Build history of the part. All positions in model axes, mm. Face numbers are marked on the shaded views. A direction names the side the tool comes from. Coordinates: 2 decimals unless noted, no trailing zeros. Loops run counter-clockwise (first coordinate to the right, second up) from the corner with the lowest first, then second, coordinate; pieces in that order, holes last.
Item 1: Cut at B-B (y = 39). List the corners of the cut face in (x, z), and give its area (3 significant figures).
Item 2: Cut at A-A (x = 39). List the corners of the cut face in (y, z), and give its area (3 significant figures).
Item 3: Flat gauge pins, fed straight in: pin 1 (8 mm diameter, centred on y = -15.5, z = 59.5, fed in from -X); pin 2 (2 mm diameter, centred on x = 15, y = 17, fed in from +Z); pin 3 (8 mm diameter, centred on x = -35.5, z = 77.5, fed in from +Y). Where does each tip first touch, or does it go through?
Item 4: Drill centre lines: line 1 along Z through (x, y) = (-13, 0); line 2 along Y through (x, z) = (-22.5, 70); line 3 along X through (y, z) = (13.5, 57.5). Where is each one in solid material? Low to high.
Item 5: 3-axis set-ups, long thin cutter, end or side, ignore diameter. For the marked faces 1, 2, 3 and 4: which of +Z, -Z, +X, -X, +Y, -Y reach the whole face in a straight line?
Item 6: Cut at C-C (z = 20.5). List the corners of the cut face in (x, y), and give its area (3 significant figures).
from build123d import *

# Parameters (mm, degrees)
F0_W      = 100
F0_H      = 100
F1_DEPTH  = 75
F2_W      = 52.5
F2_H      = 52.5
F3_DEPTH  = 10
F4_W      = 5
F4_H      = 52.5
F5_DEPTH  = 1
F6_W      = 10
F6_H      = 10
F7_DEPTH  = 1
F8_W      = 10
F8_H      = 11
F9_DEPTH  = 1
F10_W     = 10
F10_H     = 3.468894
F11_DEPTH = 1
F12_W     = 10
F12_H     = 3.531106
F13_DEPTH = 1


with BuildPart() as f1:
    # F0 (on Top) → F1 (new body)
    with BuildSketch(Plane.XY):
        with Locations((-0.019781, -0.031106)):
            Rectangle(F0_W, F0_H)
    extrude(amount=F1_DEPTH)

    # F2 (on face) → F3 (join)
    with BuildSketch(Plane.XY.offset(75)):
        with Locations((26.25, 26.25)):
            Rectangle(F2_W, F2_H)
        with Locations((-26.25, 26.25)):
            Rectangle(F2_W, F2_H)
        with Locations((26.25, -26.25)):
            Rectangle(F2_W, F2_H)
        with Locations((-26.25, -26.25)):
            Rectangle(F2_W, F2_H)
    extrude(amount=F3_DEPTH)

    # F4 (on face) → F5 (join)
    with BuildSketch(Plane.XY.offset(85)):
        with Locations((-2.5, -26.25)):
            Rectangle(F4_W, F4_H)
        with Locations((-2.5, 26.25)):
            Rectangle(F4_W, F4_H)
        with Locations((2.5, -26.25)):
            Rectangle(F4_W, F4_H)
        with Locations((2.5, 26.25)):
            Rectangle(F4_W, F4_H)
    extrude(amount=F5_DEPTH)

    # F6 (on face) → F7 (join)
    with BuildSketch(Plane.XZ.offset(52.5)):
        with Locations((0, 80)):
            Rectangle(F6_W, F6_H)
    extrude(amount=F7_DEPTH)

    # F8 (on face) → F9 (join)
    with BuildSketch(Plane(origin=(0, 52.5, 0), x_dir=(-1, 0, 0), z_dir=(0, 1, 0))):
        with Locations((0, 80.5)):
            Rectangle(F8_W, F8_H)
    extrude(amount=F9_DEPTH)

    # F10 (on face) → F11 (join)
    with BuildSketch(Plane(origin=(0, 0, 75), x_dir=(1, 0, 0), z_dir=(0, 0, -1))):
        with Locations((0, 51.765553)):
            Rectangle(F10_W, F10_H)
    extrude(amount=F11_DEPTH)

    # F12 (on face) → F13 (join)
    with BuildSketch(Plane(origin=(0, 0, 75), x_dir=(1, 0, 0), z_dir=(0, 0, -1))):
        with Locations((0, -51.734447)):
            Rectangle(F12_W, F12_H)
    extrude(amount=F13_DEPTH)


solid = f1.part
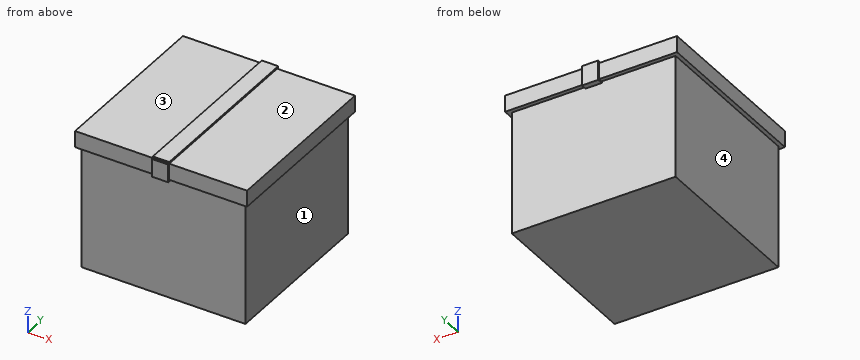
Filled sheet:
1. outline: (-52.5, 75) - (-50.02, 75) - (-50.02, 0) - (49.98, 0) - (49.98, 75) - (52.5, 75) - (52.5, 85) - (5, 85) - (5, 86) - (-5, 86) - (-5, 85) - (-52.5, 85) - close
1. area: 8,560 mm2
2. outline: (-52.5, 75) - (-50.03, 75) - (-50.03, 0) - (49.97, 0) - (49.97, 75) - (52.5, 75) - (52.5, 85) - (-52.5, 85) - close
2. area: 8,550 mm2
3. pin 1: stops at x = -50.02
3. pin 2: stops at z = 85
3. pin 3: stops at y = 52.5
4. line 1: z = 0 to 85
4. line 2: y = -50.03 to 49.97
4. line 3: x = -50.02 to 49.98
5. face 1: -Z, +X, +Y, -Y
5. face 2: +Z, +X, +Y, -Y
5. face 3: +Z, -X, +Y, -Y
5. face 4: -Z, -X, +Y, -Y
6. outline: (-50.02, -50.03) - (49.98, -50.03) - (49.98, 49.97) - (-50.02, 49.97) - close
6. area: 10,000 mm2
